For this review, take the finished solid that the model builds, in its own axes (mm). Face numbers are marked on the shaded views. Round coordinates to 2 decimals unless told otherwise and drop trailing zeros. Write each loop counter-clockwise with the first axis right and the second up, starting at its lowest first coordinate (ties: lowest second). Pieces come first, ordered by that corner, then holes. Notation, with made-up numbers: M 86,76 L 97,76 A14 ccw 97,96 Z; hole C 84,59.5 d2. An arc over 180 degrees is marked long. Use one line per item in the form item = value. Start each with the question number.
Item 1: For P1, Ø4, axis at y = 25, z = 4.5, coming from the -X side; P2, Ø1.5, axis at y = 30.5, z = 4.5, coming from the +X side, all flat-tipped, find the tip position at first contact; note any pin that passes through.
Item 2: Add section A-A (z = 9). State the section outline as (x, y) points, and give its area (3 significant figures).
Item 3: Add section D-D (x = 3). State the section outline as (y, z) points.
Item 4: Draft analysis for pull direction Z (two halves, no side actions). For the marked faces 1, 2 and 3, state which applies: released by +Z, released by -Z, zero draft, split by the parting line, or undercut.
Item 5: Add section C-C (y = -31.5). State the section outline as (x, z) points.
Item 6: For line 1 (X direction, y = -8.5, z = 7.25); line 2 (X direction, y = -41, z = 5.25); line 3 (Y direction, x = 18, z = 5.5), list the stretches that pass through material, from the lowest coordinate up. Write a range as [from, to].
Item 7: Add section B-B (x = -16). State the section outline as (y, z) points, and give its area (3 significant figures).
from build123d import *

# Parameters (mm, degrees)
SKETCH1_W           = 103.2
SKETCH1_H           = 60
BOSS_EXTRUDE1_DEPTH = 10
CUT_EXTRUDE6_DEPTH  = 108.936277497
SKETCH16_W          = 5.4
SKETCH16_H          = 5.4
CUT_EXTRUDE7_DEPTH  = 61.519087898


with BuildPart() as part:
    # Sketch1 → Boss-Extrude1 (new body)
    with BuildSketch(Plane(origin=(0, 0, 0), x_dir=(0, 1, 0), z_dir=(0, 0, 1))):
        Rectangle(SKETCH1_W, SKETCH1_H)
    extrude(amount=BOSS_EXTRUDE1_DEPTH)

    # Sketch14 → Cut-Extrude6 (cut, through all)
    with BuildSketch(Plane(origin=(0, 51.6, 0), x_dir=(-1, 0, 0), z_dir=(0, 1, 0))):
        Polygon((-30, 6.5), (-27.2, 6.5), (-27.2, 8), (-24.7, 8), (-24.7, 6), (-24.7, 3), (-30, 3), align=None)
        Polygon((30, 6.5), (30, 3), (24.7, 3), (24.7, 6), (24.7, 8), (27.2, 8), (27.2, 6.5), align=None)
        Polygon((17.95, 8), (7.55, 8), (7.55, 10), (-7.55, 10), (-7.55, 8), (-17.95, 8), (-17.95, 5.6), (17.95, 5.6), align=None)
    extrude(amount=-CUT_EXTRUDE6_DEPTH, mode=Mode.SUBTRACT)

    # Sketch16 → Cut-Extrude7 (cut, through all)
    with BuildSketch(Plane.XY.offset(10)):
        with Locations((17.35, -41.9)):
            Rectangle(SKETCH16_W, SKETCH16_H)
        with Locations((17.35, 41.9)):
            Rectangle(SKETCH16_W, SKETCH16_H)
        with Locations((-17.35, 41.9)):
            Rectangle(SKETCH16_W, SKETCH16_H)
        with Locations((-17.35, -41.9)):
            Rectangle(SKETCH16_W, SKETCH16_H)
    extrude(amount=-CUT_EXTRUDE7_DEPTH, mode=Mode.SUBTRACT)


solid = part.part
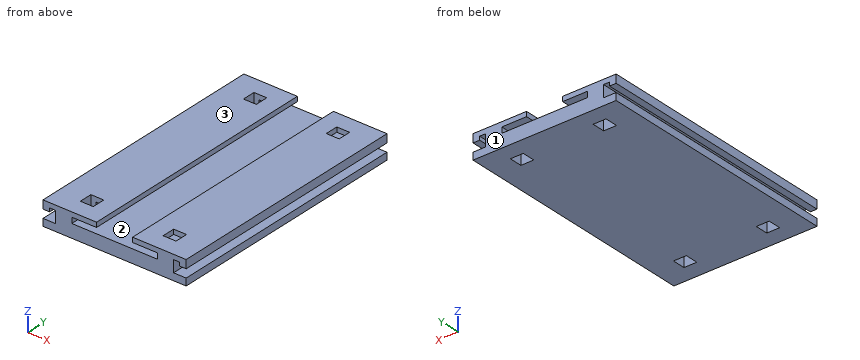
Calculated:
q1.P1 = -30
q1.P2 = 24.7
q2.outline = M -30,-51.6 L -7.55,-51.6 L -7.55,51.6 L -30,51.6 Z; M 7.55,-51.6 L 30,-51.6 L 30,51.6 L 7.55,51.6 Z; hole M -20.05,-44.6 L -14.65,-44.6 L -14.65,-39.2 L -20.05,-39.2 Z; hole M -20.05,39.2 L -14.65,39.2 L -14.65,44.6 L -20.05,44.6 Z; hole M 14.65,-44.6 L 20.05,-44.6 L 20.05,-39.2 L 14.65,-39.2 Z; hole M 14.65,39.2 L 20.05,39.2 L 20.05,44.6 L 14.65,44.6 Z
q2.area = 4,520 mm^2
q3.outline = M -51.6,0 L 51.6,0 L 51.6,5.6 L -51.6,5.6 Z
q4.face_1 = zero draft
q4.face_2 = undercut
q4.face_3 = released by +Z
q5.outline = M -30,0 L 30,0 L 30,3 L 24.7,3 L 24.7,8 L 27.2,8 L 27.2,6.5 L 30,6.5 L 30,10 L 7.55,10 L 7.55,8 L 17.95,8 L 17.95,5.6 L -17.95,5.6 L -17.95,8 L -7.55,8 L -7.55,10 L -30,10 L -30,6.5 L -27.2,6.5 L -27.2,8 L -24.7,8 L -24.7,3 L -30,3 Z
q6.line_1 = [-30, -27.2], [-24.7, -17.95], [17.95, 24.7], [27.2, 30]
q6.line_2 = [-24.7, -20.05], [-14.65, 14.65], [20.05, 24.7]
q6.line_3 = [-51.6, -44.6], [-39.2, 39.2], [44.6, 51.6]
q7.outline = M -51.6,0 L -44.6,0 L -44.6,5.6 L -51.6,5.6 Z; M -51.6,8 L -44.6,8 L -44.6,10 L -51.6,10 Z; M -39.2,0 L 39.2,0 L 39.2,5.6 L -39.2,5.6 Z; M -39.2,8 L 39.2,8 L 39.2,10 L -39.2,10 Z; M 44.6,0 L 51.6,0 L 51.6,5.6 L 44.6,5.6 Z; M 44.6,8 L 51.6,8 L 51.6,10 L 44.6,10 Z
q7.area = 702 mm^2
